from build123d import *

# Parameters (mm, degrees)
F1_DEPTH  = 63.5
F2_W      = 31.75
F2_H      = 12.7
F2_W_2    = 6.35
F2_H_2    = 20.0227687303
F3_DEPTH  = 6.35
F4_W      = 38.1
F4_H      = 6.35
F5_DEPTH  = 74.629437754
F7_DEPTH  = 74.629437754
F8_R      = 14.2875
F8_R_2    = 6.7437
F9_DEPTH  = 9.2456
F10_R     = 6.7437
F11_DEPTH = 23.4781687303
F12_W     = 31.75
F12_H     = 12.7
F13_DEPTH = 6.35


with BuildPart() as f1:
    # F0 (on Front) → F1 (new body)
    with BuildSketch(Plane.XZ):
        Polygon((0, 43.474850689), (0, 0), (61.928437754, 0), (61.928437754, -20.0227687303), (74.628437754, -20.0227687303), (74.628437754, 12.7), (61.928437754, 12.7), (30.178437754, 12.7), (12.7, 12.7), (12.7, 43.474850689), align=None)
    extrude(amount=F1_DEPTH)

    # F2 (on face) → F3 (cut, symmetric)
    with BuildSketch(Plane.XZ.offset(63.5)):
        with Locations((43.3283648044, 6.35)):
            Rectangle(F2_W, F2_H)
        with Locations((65.103437754, -10.0113843652)):
            Rectangle(F2_W_2, F2_H_2)
    extrude(amount=F3_DEPTH, both=True, mode=Mode.SUBTRACT)

    # F4 (on face) → F5 (cut, through all)
    with BuildSketch(Plane.YZ.offset(74.628437754)):
        with Locations((-31.75, -16.8477687303)):
            Rectangle(F4_W, F4_H)
    extrude(amount=-F5_DEPTH, mode=Mode.SUBTRACT)

    # F6 (on Right) → F7 (cut, through all)
    with BuildSketch(Plane.YZ):
        with BuildLine():
            Line((-21.9217978256, 37.9429917058), (-45.1858863235, 37.9429917058))
            ThreePointArc((-45.1858863235, 37.9429917058), (-53.0598863235, 30.0689917058), (-45.1858863235, 22.1949917058))
            Line((-45.1858863235, 22.1949917058), (-21.9217978256, 22.1949917058))
            ThreePointArc((-21.9217978256, 22.1949917058), (-14.0477978256, 30.0689917058), (-21.9217978256, 37.9429917058))
        make_face()
    extrude(amount=F7_DEPTH, mode=Mode.SUBTRACT)

    # F8 (on face) → F9 (cut)
    with BuildSketch(Plane.XY.offset(12.7)):
        with Locations((43.3283648044, -31.9399088621)):
            Circle(F8_R)
        with Locations((43.3283648044, -31.9399088621)):
            Circle(F8_R_2, mode=Mode.SUBTRACT)
        with Locations((43.3283648044, -31.9399088621)):
            Circle(F8_R_2)
    extrude(amount=-F9_DEPTH, mode=Mode.SUBTRACT)

    # F10 (on face) → F11 (cut, through all)
    with BuildSketch(Plane.XY.offset(3.4544)):
        with Locations((43.3283648044, -31.9399088621)):
            Circle(F10_R)
    extrude(amount=-F11_DEPTH, mode=Mode.SUBTRACT)

    # F12 (on face) → F13 (cut, symmetric)
    with BuildSketch(Plane(origin=(0, 0, 0), x_dir=(-1, 0, 0), z_dir=(0, 1, 0))):
        with Locations((-46.053437754, 6.35)):
            Rectangle(F12_W, F12_H)
    extrude(amount=F13_DEPTH, both=True, mode=Mode.SUBTRACT)


solid = f1.part
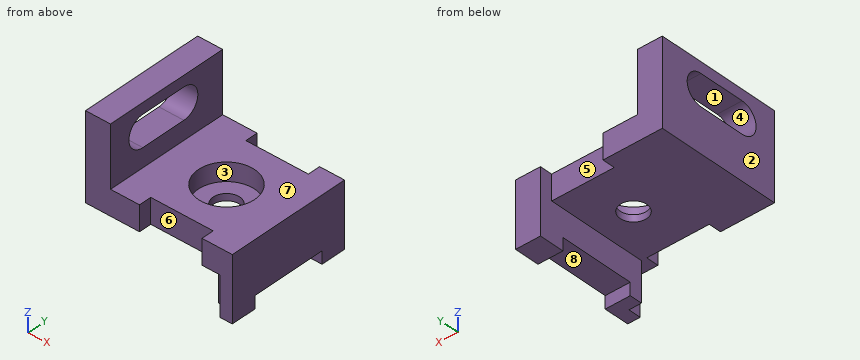
Read the model definition and answer for the solid it produces. Units are mm, in the model's axes. Face numbers are marked on the shaded views. A direction names the side the tool comes from. Coordinates: 2 decimals unless noted, no trailing zeros. Loops run counter-clockwise (first coordinate to the right, second up) from the corner with the lowest first, then second, coordinate; pieces in that order, holes last. Notation, with made-up numbers: (51, 69.25) - (62, 69.25) arc R20 cw to (62, 81.25) - close; hole circle Ø7 at (33, -19). An arc over 180 degrees is marked (long way). Answer in a Markdown table with one row per item.
Q1. For the marked faces 4, 5, 6, 7 and 8, determine the directions among +Z, -Z, +X, -X, +Y, -Y from which every point of the face is accessible in a straight line to the end or side of a thin tool.
Here are the results:
| item | result |
|---|---|
| face 4 | +X, -X |
| face 5 | +Z, -Z, +Y |
| face 6 | +Z, -Z, -Y |
| face 7 | +Z, +X, +Y, -Y |
| face 8 | -Z, +X, -X |
Q2. The mould has two halves that part along X. Classify the marked faces 1, 2 and 3: pulls with the +X half, pulls with the -X half, needs draft (parallel to the pull), parting line crosses it, or undercut.
Here are the results:
| item | result |
|---|---|
| face 1 | needs draft |
| face 2 | pulls with the -X half |
| face 3 | undercut |
Q3. Find section D-D on y = -10. Write down the section's boundary in (x, z).
Here are the results:
| item | result |
|---|---|
| outline | (0, 0) - (61.93, 0) - (61.93, -20.02) - (74.63, -20.02) - (74.63, 12.7) - (12.7, 12.7) - (12.7, 43.47) - (0, 43.47) - close |
Q4. Straight lines are drawn through the part: line 1 along Z through (x, y) = (27.5, -25); line 2 along X through (y, z) = (-32, -6). For each, find the intervals that lie inside material, in ascending order. Write a range as [from, to].
Here are the results:
| item | result |
|---|---|
| line 1 | z = [0, 12.7] |
| line 2 | x = [61.93, 74.63] |
Q5. Find section A-A on x = 46. Write down the section's boundary in (y, z).
Here are the results:
| item | result |
|---|---|
| outline | (-57.15, 0) - (-38.13, 0) - (-38.13, 3.45) - (-45.98, 3.45) - (-45.98, 12.7) - (-57.15, 12.7) - close; (-25.75, 0) - (-6.35, 0) - (-6.35, 12.7) - (-17.9, 12.7) - (-17.9, 3.45) - (-25.75, 3.45) - close |
Q6. Given P1, Ø24.5, axis at y = -32.5, z = 35.5, coming from the +X side; P2, Ø7, axis at y = -62, z = -13, coming from the -X side; P3, Ø14, axis at x = 53.5, z = 6, coming from the +Y side, each flat-ended and moving along its own axis, determine where each tip first touches the part or whether it passes through.
Here are the results:
| item | result |
|---|---|
| P1 | stops at x = 12.7 |
| P2 | stops at x = 68.28 |
| P3 | stops at y = -6.35 |
Q7. Find section B-B on y = -34. Write down the section's boundary in (x, z) (3 decimals).
Here are the results:
| item | result |
|---|---|
| outline | (0, 0) - (36.907, 0) - (36.907, 3.454) - (29.19, 3.454) - (29.19, 12.7) - (12.7, 12.7) - (12.7, 22.195) - (0, 22.195) - close; (0, 37.943) - (12.7, 37.943) - (12.7, 43.475) - (0, 43.475) - close; (49.75, 0) - (61.928, 0) - (61.928, -13.673) - (74.628, -13.673) - (74.628, 12.7) - (57.467, 12.7) - (57.467, 3.454) - (49.75, 3.454) - close |
Q8. Find section C-C on z = 32. Write down the section's boundary in (x, y), plus the area to 3 significant figures.
Here are the results:
| item | result |
|---|---|
| outline | (0, -63.5) - (12.7, -63.5) - (12.7, -52.82) - (0, -52.82) - close; (0, -14.29) - (12.7, -14.29) - (12.7, 0) - (0, 0) - close |
| area | 317 mm^2 |
